from build123d import *

# Parameters (mm, degrees)
SKETCH4_R          = 19.05
CUT_EXTRUDE3_DEPTH = 113.506231401
SKETCH6_R          = 7.1501
CUT_EXTRUDE5_DEPTH = 113.506231401
CIRPATTERN2_COUNT  = 4
FILLET1_R          = 4.826


with BuildPart() as part:
    # Sketch1 → Revolve1 (revolve)
    with BuildSketch(Plane.XY, mode=Mode.PRIVATE) as revolve1_sk:
        Polygon((-36.322, 35.052), (-1.524, 35.052), (-1.524, 0), (-55.372, 0), (-55.372, 69.85), (-36.322, 69.85), align=None)
    revolve(revolve1_sk.sketch.rotate(Axis((-88.771392405, 0, 0), (1, 0, 0)), 90), axis=Axis((-88.771392405, 0, 0), (1, 0, 0)))

    # Sketch4 → Cut-Extrude3 (cut, through all)
    with BuildSketch(Plane.ZY.offset(55.372)):
        Circle(SKETCH4_R)
    extrude(amount=-CUT_EXTRUDE3_DEPTH, mode=Mode.SUBTRACT)

    # Sketch6 → Cut-Extrude5 (cut, through all)
    with BuildSketch(Plane.ZY.offset(55.372)):
        with Locations((0, 54.082681536)):
            Circle(SKETCH6_R)
    cut_extrude5 = extrude(amount=-CUT_EXTRUDE5_DEPTH, mode=Mode.SUBTRACT)

    # CirPattern2: Cut-Extrude5 ×4 about axis
    cirpattern2_axis = Axis((0, 0, 0), (1, 0, 0))
    for i in range(1, CIRPATTERN2_COUNT):
        add(cut_extrude5.rotate(cirpattern2_axis, i * 360 / CIRPATTERN2_COUNT), mode=Mode.SUBTRACT)

    # Fillet1
    fillet1_edges = [part.edges().sort_by_distance(p)[0] for p in [
        (-36.322, 0, -35.052),
        (-1.524, 0, -35.052),
        (-36.322, 0, -69.85),
    ]]
    fillet(fillet1_edges, radius=FILLET1_R)


solid = part.part
Input: part model. Units: mm. Frame: model coordinates. Round coordinates to 2 decimals unless told otherwise and drop trailing zeros. Order: outer loops, then holes, each group sorted by start corner. A loop starts at its lowest first (then second) coordinate and runs counter-clockwise, first axis right, second up. Notation, with made-up numbers: (-33.75, 39) - (10.25, 39) arc R7 cw to (10.25, 45) - close; hole circle Ø9 at (77.5, -23). An arc over 180 degrees is marked (long way). Use a Markdown table: item, result.
1. First-contact query: pin 1 (1.5 mm diameter, centred on x = -24.5, z = -14.5, fed in from +Y); pin 2 (8.5 mm diameter, centred on y = 0, z = -54.08, fed in from -X); pin 3 (3 mm diameter, centred on x = -32, y = -11, fed in from +Z); pin 4 (4 mm diameter, centred on x = -12, z = -5.5, fed in from -Y). Flat tips, straight axial feed; report the tip coordinate or a pass-through.
Evaluation:
| item | result |
|---|---|
| pin 1 | y = 32.24 |
| pin 2 | through |
| pin 3 | z = 33.89 |
| pin 4 | y = -34.88 |
2. Material intervals for probe 1 along Y at (x, z) = (-44.5, 0); probe 2 along X at (y, z) = (30.5, -48.5); probe 3 along Z at (x, y) = (-38, 9.5), sorted ascending.
Evaluation:
| item | result |
|---|---|
| probe 1 | -69.85 to -61.23, -46.93 to -19.05, 19.05 to 46.93, 61.23 to 69.85 |
| probe 2 | -55.37 to -36.32 |
| probe 3 | -68.02 to -16.51, 16.51 to 68.02 |
3. Mould query, pull axis Y, two halves, no side actions, for faces 1 (the face through (-18.747, -10.529, 33.433)), 2 (the face through (-28.82, -11.59, -15.12)), 3 (the face through (-36.322, 28, -30)). Classes: +Y half, -Y half, draft (parallel to the pull), parting line (faces both ways), or undercut.
Evaluation:
| item | result |
|---|---|
| face 1 | parting line |
| face 2 | undercut |
| face 3 | draft |
4. Section D-D on x = -43. Return the cut outline in (y, z), then the cut area to 3 significant figures.
Evaluation:
| item | result |
|---|---|
| outline | circle Ø139.7 at (0, 0); hole circle Ø14.3 at (-54.08, 0); hole circle Ø38.1 at (0, 0); hole circle Ø14.3 at (0, -54.08); hole circle Ø14.3 at (0, 54.08); hole circle Ø14.3 at (54.08, 0) |
| area | 13,500 mm^2 |
5. Section C-C on x = -23.5. Return the cut outline in (y, z).
Evaluation:
| item | result |
|---|---|
| outline | circle Ø70.1 at (0, 0); hole circle Ø38.1 at (0, 0) |
6. Section A-A on z = 0. Return the cut outline in (x, y), then the cut area to 3 significant figures.
Evaluation:
| item | result |
|---|---|
| outline | (-55.37, -69.85) - (-41.15, -69.85) arc R4.83 ccw to (-36.32, -65.02) - (-36.32, -61.23) - (-55.37, -61.23) - close; (-55.37, -46.93) - (-36.32, -46.93) - (-36.32, -39.88) arc R4.83 cw to (-31.5, -35.05) - (-6.35, -35.05) arc R4.83 ccw to (-1.52, -30.23) - (-1.52, -19.05) - (-55.37, -19.05) - close; (-55.37, 19.05) - (-1.52, 19.05) - (-1.52, 30.23) arc R4.83 ccw to (-6.35, 35.05) - (-31.5, 35.05) arc R4.83 cw to (-36.32, 39.88) - (-36.32, 46.93) - (-55.37, 46.93) - close; (-55.37, 61.23) - (-36.32, 61.23) - (-36.32, 65.02) arc R4.83 ccw to (-41.15, 69.85) - (-55.37, 69.85) - close |
| area | 2,490 mm^2 |
